from build123d import *

# Parameters (mm, degrees)
F1_DEPTH = 1800
F2_R     = 3.25
F3_DEPTH = 25


with BuildPart() as f1:
    # F0 (on Right) → F1 (new body)
    with BuildSketch(Plane.YZ):
        Polygon((0, 62), (0, 0), (62, 0), (62, 20), (60, 20), (60, 2), (2, 2), (2, 62), align=None)
    extrude(amount=-F1_DEPTH)

    # F2 (on face) → F3 (cut)
    with BuildSketch(Plane(origin=(0, 2, 0), x_dir=(-1, 0, 0), z_dir=(0, 1, 0))):
        with Locations((20, 47)):
            Circle(F2_R)
        with Locations((50, 47)):
            Circle(F2_R)
        with Locations((20, 17)):
            Circle(F2_R)
        with Locations((50, 17)):
            Circle(F2_R)
        with Locations((1750, 47)):
            Circle(F2_R)
        with Locations((1780, 47)):
            Circle(F2_R)
        with Locations((1780, 17)):
            Circle(F2_R)
        with Locations((1750, 17)):
            Circle(F2_R)
    extrude(amount=-F3_DEPTH, mode=Mode.SUBTRACT)


solid = f1.part
Source: CAD feature listing. Evaluate the final solid. Frame: model axes, mm. A direction names the side the tool comes from. Coordinates: 2 decimals unless noted, no trailing zeros. Loops run counter-clockwise (first coordinate to the right, second up) from the corner with the lowest first, then second, coordinate; pieces in that order, holes last. Notation, with made-up numbers: M 60,42.25 L 95,42.25 A21 cw 95,48.25 Z; hole C -29,85 d3. An arc over 180 degrees is marked long. Answer in a Markdown table with one row per item.
Q1. Set-up query: faces 4 (the flat face through (-887, 0, 31)), 5 (the flat face through (-887, 2, 32)). Return all of +Z, -Z, +X, -X, +Y, -Y with unobstructed straight access to the full face (end or side cutting, diameter ignored); none if empty.
Answers below:
| item | result |
|---|---|
| face 4 | +Z, -Z, +X, -X, -Y |
| face 5 | +Z, +X, -X |
Q2. Section B-B on y = 48. Return the cut outline in (x, z).
Answers below:
| item | result |
|---|---|
| outline | M -1800,0 L 0,0 L 0,2 L -1800,2 Z |
Q3. Section A-A on x = -628. Return the cut outline in (y, z), plus the area to 3 significant figures.
Answers below:
| item | result |
|---|---|
| outline | M 0,0 L 62,0 L 62,20 L 60,20 L 60,2 L 2,2 L 2,62 L 0,62 Z |
| area | 280 mm^2 |
Q4. Draft query along X for faces 1 (the flat face through (0, 22, 1)), 2 (the flat face through (-887, 31, 2)), 3 (the flat face through (-1800, 22, 1)). Return one class per face: pulls with the +X half, pulls with the -X half, needs draft (parallel to the pull), parting line crosses it, or undercut.
Answers below:
| item | result |
|---|---|
| face 1 | pulls with the +X half |
| face 2 | needs draft |
| face 3 | pulls with the -X half |
Q5. Ray query, probe 1 along Z at (x, y) = (-20, 1); probe 2 along Y at (x, z) = (-870, 18); probe 3 along Z at (x, y) = (-828.5, 7.5). Return the intervals inside material, ascending. Write a range as from..to.
Answers below:
| item | result |
|---|---|
| probe 1 | z = 0..13.75, 20.25..43.75, 50.25..62 |
| probe 2 | y = 0..2, 60..62 |
| probe 3 | z = 0..2 |
Q6. First-contact query: pin 1 (20 mm diameter, centred on x = -599, z = 12.5, fed in from -Y); pin 2 (6 mm diameter, centred on x = -1210.5, z = 40, fed in from +Y); pin 3 (5 mm diameter, centred on x = -347.5, y = 47.5, fed in from +Z); pin 4 (12 mm diameter, centred on x = -423.5, y = 55.5, fed in from +Z). Flat tips, straight axial feed; report the tip coordinate or a pass-through.
Answers below:
| item | result |
|---|---|
| pin 1 | stops at y = 0 |
| pin 2 | stops at y = 2 |
| pin 3 | stops at z = 2 |
| pin 4 | stops at z = 20 |
